Geometry: final body of the model. Coordinates: model frame, mm. Face numbers are marked on the shaded views. A direction names the side the tool comes from. Round coordinates to 2 decimals unless told otherwise and drop trailing zeros. Write each loop counter-clockwise with the first axis right and the second up, starting at its lowest first coordinate (ties: lowest second). Pieces come first, ordered by that corner, then holes. Notation, with made-up numbers: M 88.25,-20 L 124.25,-20 A26 ccw 124.25,-5 Z; hole C -7,-32 d3. An arc over 180 degrees is marked long. Answer as CSV lines item,"result". Start each with the question number.
Q1. Section query D-D on x = 0. Give the number of separate pieces and of enclosed holes in the cut face, and give its area (3 significant figures).
Q2. First-contact query: pin 1 (5 mm diameter, centred on x = -0.5, z = 14.5, fed in from +Y); pin 2 (12 mm diameter, centred on x = -4.5, z = -2, fed in from +Y). Flat tips, straight axial feed; report the tip coordinate or a pass-through.
Q3. Section query B-B on z = 13. Output: boundary loops of the cut face in (x, y), and give its area (3 significant figures).
Q4. Section query C-C on y = 50. Output: boundary loops of the cut face in (x, z) (3 decimals).
Q5. Mould query, pull axis Z, two halves, no side actions, for the marked faces 1, 2, 3 and 4. Classes: pulls with the +Z half, pulls with the -Z half, needs draft (parallel to the pull), parting line crosses it, or undercut.
Q6. Reachability of the marked faces 5 and 6 from +Z, -Z, +X, -X, +Y, -Y: full face, straight path, thin tool, end or side. Return the list, or none.
Q7. Ray query, probe 1 along Z at (x, y) = (0, 4.75) (3 decimals); probe 2 along Y at (x, z) = (0, -29); probe 3 along X at (y, z) = (-2.25, 13). Return the intervals inside material, ascending.
Q8. Section query A-A on y = 37.5. Output: boundary loops of the cut face in (x, z) (3 decimals).
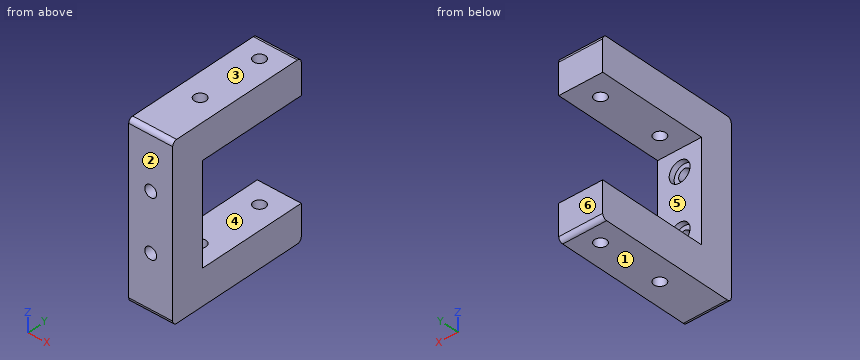
Autodesk Inventor part; units mm, degrees
ref_plane "YZ Plane" through (0, 0, 0) normal (1, 0, 0) x (0, 1, 0)
ref_plane "XZ Plane" through (0, 0, 0) normal (0, 1, 0) x (-1, 0, 0)
ref_plane "XY Plane" through (0, 0, 0) normal (0, 0, 1) x (1, 0, 0)
sketch "Boceto1" plane through (0, 0, 0) normal (0, 1, 0) x (-1, 0, 0)
  line L0 (-6.45, 25.5) -> (6.45, 25.5)
  line L1 (6.45, 25.5) -> (6.45, -25.5)
  line L2 (6.45, -25.5) -> (-6.45, -25.5)
  line L3 (-6.45, -25.5) -> (-6.45, 25.5)
  line L4 (-6.45, 25.5) -> (6.45, -25.5) construction
  line L5 (6.45, 25.5) -> (-6.45, -25.5) construction
  circle A0 centre (0, 0) radius 3.5
  dimension "d0" = 7
  dimension "d1" = 51
  dimension "d2" = 12.9
extrude "Extrusión1" add sketch "Boceto1" along normal blind 10
sketch "Boceto2" plane through (0, 10, 0) normal (0, 1, 0) x (1, 0, 0)
  circle A0 centre (0, 0) radius 6
  dimension "d5" = 12
extrude "Extrusión2" cut sketch "Boceto2" against normal blind 6
sketch "Boceto3" plane through (0, 10, 0) normal (0, 1, 0) x (1, 0, 0)
  circle A0 centre (0, 0) radius 6
  line L0 (6.45, 25.5) -> (-6.45, 25.5)
  line L1 (-6.45, 25.5) -> (-6.45, -25.5)
  line L2 (-6.45, -25.5) -> (6.45, -25.5)
  line L3 (6.45, -25.5) -> (6.45, 25.5)
  line L4 (10, -38.575) -> (-10, -38.575)
  line L5 (-10, -38.575) -> (-10, 38.575)
  line L6 (-10, 38.575) -> (10, 38.575)
  line L7 (10, 38.575) -> (10, -38.575)
  line L8 (10, -38.575) -> (-10, 38.575) construction
  line L9 (-10, -38.575) -> (10, 38.575) construction
  dimension "d21" = 20
  dimension "d22" = 77.15
extrude "Extrusión3" add sketch "Boceto3" against normal blind 15 contours L4 L5 L6 L7
sketch "Boceto4" plane through (0, 10, 0) normal (0, 1, 0) x (1, 0, 0)
  line L0 (10, -38.575) -> (-10, -38.575)
  line L1 (10, -38.575) -> (10, 38.575)
  line L2 (-10, -38.575) -> (10, -38.575)
  line L3 (10, -38.575) -> (10, -22.575)
  line L4 (10, -22.575) -> (-10, -22.575)
  line L5 (-10, -22.575) -> (-10, -38.575)
  line L6 (10, 38.575) -> (-10, 38.575)
  line L7 (-10, 38.575) -> (10, 38.575)
  line L8 (10, 38.575) -> (10, 22.575)
  line L9 (10, 22.575) -> (-10, 22.575)
  line L10 (-10, 22.575) -> (-10, 38.575)
  point P0 (0, 0)
  point P1 (10, 22.575)
  dimension "d12" = 16
  dimension "d13" = 16
extrude "Extrusión4" add sketch "Boceto4" along normal blind 50
sketch "Boceto5" plane through (-10, -5, 38.575) normal (0, 0, 1) x (1, 0, 0)
  circle A0 centre (10, 55) radius 2.7
  circle A1 centre (10, 25) radius 2.6954
  line L0 (0, 65) -> (20, 65)
  point P0 (10, 5)
  point P1 (20, 15)
  dimension "d16" = 5.4
  dimension "d17" = 10
  dimension "d18" = 10
extrude "Extrusión5" cut sketch "Boceto5" against normal through all
sketch "Boceto6" plane through (0, 10, 0) normal (0, 1, 0) x (1, 0, 0)
  circle A0 centre (0, 0) radius 6
extrude "Extrusión6" add sketch "Boceto6" against normal up to surface (10 mm away)
sketch "Boceto7" plane through (0, -5, 0) normal (0, -1, 0) x (1, 0, 0)
  line L0 (-10, -38.575) -> (10, -38.575)
  line L1 (10, -38.575) -> (10, 38.575)
  line L2 (10, 38.575) -> (-10, 38.575)
  line L3 (-10, 38.575) -> (-10, -38.575)
  line L4 (6.45, 25.5) -> (6.45, -25.5)
  line L5 (6.45, -25.5) -> (-6.45, -25.5)
  line L6 (-6.45, -25.5) -> (-6.45, 25.5)
  line L7 (-6.45, 25.5) -> (6.45, 25.5)
  line L8 (6.45, -25.5) -> (-6.45, -25.5)
  line L9 (6.45, 25.5) -> (6.45, -25.5)
  line L10 (-6.45, 25.5) -> (6.45, 25.5)
  line L11 (-6.45, -25.5) -> (-6.45, 25.5)
  point P0 (0, 0)
extrude "Extrusión7" add sketch "Boceto7" against normal up to surface (5 mm away) contours L4 L5 L6 L7
sketch "Boceto8" plane through (0, 10, 0) normal (0, 1, 0) x (1, 0, 0)
  circle A0 centre (0, -13) radius 2.7
  circle A1 centre (0, 13) radius 2.7
  point P0 (0, 0)
  dimension "d27" = 5.4
  dimension "d28" = 13
  dimension "d29" = 13
extrude "Extrusión8" cut sketch "Boceto8" against normal through all
sketch "Boceto9" plane through (0, 10, 0) normal (0, 1, 0) x (1, 0, 0)
  circle A0 centre (0, -13) radius 2.7
  circle A1 centre (0, -13) radius 4.75
  circle A2 centre (0, 13) radius 2.7
  circle A3 centre (0, 13) radius 4.75
  point P0 (0, 0)
  dimension "d32" = 9.5
  dimension "d33" = 9.5
extrude "Extrusión9" cut sketch "Boceto9" against normal blind 2.5
fillet "Empalme1" radius 2 4 edges at (0, -5, 38.575) (0, 60, 38.575) (0, 60, -38.575) (0, -5, -38.575)
properties part number "LowerJaw"
Entries:
1,separate pieces,"7"
1,enclosed holes,"0"
1,area,"2,230 mm^2"
2,pin 1,"stops at y = 7.5"
2,pin 2,"stops at y = 10"
3,outline,"M -10,-5 L -2.7,-5 L -2.7,7.5 L -4.75,7.5 L -4.75,10 L -10,10 Z; M 2.7,-5 L 10,-5 L 10,10 L 4.75,10 L 4.75,7.5 L 2.7,7.5 Z"
3,area,"209 mm^2"
4,outline,"M -10,-38.575 L -2.7,-38.575 L -2.7,-22.575 L -10,-22.575 Z; M -10,22.575 L -2.7,22.575 L -2.7,38.575 L -10,38.575 Z; M 2.7,-38.575 L 10,-38.575 L 10,-22.575 L 2.7,-22.575 Z; M 2.7,22.575 L 10,22.575 L 10,38.575 L 2.7,38.575 Z"
5,face 1,"pulls with the -Z half"
5,face 2,"needs draft"
5,face 3,"pulls with the +Z half"
5,face 4,"undercut"
6,face 5,"+X, -X, +Y"
6,face 6,"+Z, -Z, +X, -X, +Y"
7,probe 1,"z = -38.575 to -15.7, -10.3 to 10.3, 15.7 to 38.575"
7,probe 2,"y = -5 to 17.3, 22.7 to 47.3, 52.7 to 60"
7,probe 3,"x = -10 to -2.7, 2.7 to 10"
8,outline,"M -10,-38.575 L 10,-38.575 L 10,-22.575 L -10,-22.575 Z; M -10,22.575 L 10,22.575 L 10,38.575 L -10,38.575 Z"
